Autodesk Fusion 360 part; units mm, degrees
sketch "Sketch1" plane through (0, 0, 0) normal (0, 0, 1) x (1, 0, 0)
  line L0 (-16.25, 11.25) -> (16.25, 11.25)
  line L1 (16.25, 11.25) -> (16.25, -11.25)
  line L2 (16.25, -11.25) -> (-16.25, -11.25)
  line L3 (-16.25, -11.25) -> (-16.25, 11.25)
  line L4 (-22.25, 13.25) -> (22.25, 13.25)
  line L5 (22.25, 13.25) -> (22.25, -13.25)
  line L6 (22.25, -13.25) -> (-22.25, -13.25)
  line L7 (-22.25, -13.25) -> (-22.25, 13.25)
  line L8 (-22.25, 13.25) -> (22.25, -13.25) construction
  line L9 (22.25, 13.25) -> (-22.25, -13.25) construction
  line L10 (-19.25, 7.5) -> (-19.25, -7.5) construction
  line L11 (-22.25, 0) -> (-16.25, 0) construction
  line L12 (16.25, 0) -> (22.25, 0) construction
  line L13 (19.25, 7.5) -> (19.25, -7.5) construction
  circle A0 centre (-19.25, 7.5) radius 1
  circle A1 centre (-19.25, -7.5) radius 1
  circle A2 centre (19.25, -7.5) radius 1
  circle A3 centre (19.25, 7.5) radius 1
  point P0 (-19.25, 0)
  point P1 (-19.25, 0)
  point P2 (19.25, 0)
  point P3 (19.25, 0)
  dimension "d1" = 32.5
  dimension "d2" = 22.5
  dimension "d3" = 2
  dimension "d4" = 6
  dimension "d21" = 6
  dimension "d22" = 2
  dimension "d23" = 15
  dimension "d24" = 2
extrude "Extrude1" add sketch "Sketch1" against normal blind 2 contours L0 L1 L2 L3 | L4 L5 L6 L7
extrude "Extrude2" add sketch "Sketch1" along normal blind 10
sketch "Sketch2" plane through (0, 0, 0) normal (0, 0, 1) x (-1, 0, 0)
  line L0 (-16.25, 11.25) -> (-16.25, -11.25)
  line L1 (-16.25, -11.25) -> (16.25, -11.25)
  line L2 (16.25, -11.25) -> (16.25, 11.25)
  line L3 (16.25, 11.25) -> (-16.25, 11.25)
  line L4 (12.5, 9) -> (12.5, -9) construction
  line L5 (12.5, -9) -> (-9.5, -9) construction
  line L6 (-9.5, 9) -> (12.5, 9) construction
  line L7 (-9.5, -9) -> (-9.5, 9) construction
  line L8 (12.5, -9) -> (-9.5, 9) construction
  line L9 (12.5, 9) -> (-9.5, -9) construction
  line L10 (14.375, -11.25) -> (10.625, -11.25)
  line L11 (10.625, -11.25) -> (10.625, -6.75)
  line L12 (10.625, -6.75) -> (14.375, -6.75)
  line L13 (14.375, -6.75) -> (14.375, -11.25)
  line L14 (14.375, -11.25) -> (10.625, -6.75) construction
  line L15 (10.625, -11.25) -> (14.375, -6.75) construction
  line L16 (-7.625, -11.25) -> (-11.375, -11.25)
  line L17 (-11.375, -11.25) -> (-11.375, -6.75)
  line L18 (-11.375, -6.75) -> (-7.625, -6.75)
  line L19 (-7.625, -6.75) -> (-7.625, -11.25)
  line L20 (-7.625, -11.25) -> (-11.375, -6.75) construction
  line L21 (-11.375, -11.25) -> (-7.625, -6.75) construction
  line L22 (14.375, 11.25) -> (10.625, 11.25)
  line L23 (10.625, 11.25) -> (10.625, 6.75)
  line L24 (10.625, 6.75) -> (14.375, 6.75)
  line L25 (14.375, 6.75) -> (14.375, 11.25)
  line L26 (14.375, 11.25) -> (10.625, 6.75) construction
  line L27 (10.625, 11.25) -> (14.375, 6.75) construction
  line L28 (-11.375, 11.25) -> (-7.625, 11.25)
  line L29 (-7.625, 11.25) -> (-7.625, 6.75)
  line L30 (-7.625, 6.75) -> (-11.375, 6.75)
  line L31 (-11.375, 6.75) -> (-11.375, 11.25)
  line L32 (-11.375, 11.25) -> (-7.625, 6.75) construction
  line L33 (-7.625, 11.25) -> (-11.375, 6.75) construction
  circle A0 centre (12.5, -9) radius 0.875
  circle A1 centre (-9.5, -9) radius 0.875
  circle A2 centre (-9.5, 9) radius 0.875
  circle A3 centre (12.5, 9) radius 0.875
  circle A4 centre (-9.5, 0) radius 4.5
  point P0 (1.5, 0)
  point P1 (12.5, -9)
  point P2 (-9.5, -9)
  point P3 (12.5, 9)
  point P4 (-9.5, 9)
  dimension "d9" = 18
  dimension "d10" = 22
  dimension "d11" = 1.5
  dimension "d12" = 3.75
  dimension "d13" = 1.75
  dimension "d16" = 9
extrude "Extrude3" add sketch "Sketch2" along normal blind 7 contours L3 L28 L29 L30 L31 | L1 L16 L17 L18 L19 | L3 L22 L23 L24 L25 | L1 L10 L11 L12 L13 | A0 | A1 | A2 | A3
extrude "Extrude4" cut sketch "Sketch2" against normal through all contours A4
sketch "Sketch3" plane through (0, 0, -2) normal (0, 0, -1) x (1, 0, 0)
  circle A0 centre (9.5, 0) radius 4.5
  circle A1 centre (19.25, -7.5) radius 1
  circle A2 centre (-19.25, 7.5) radius 1
  circle A3 centre (19.25, 7.5) radius 1
  circle A4 centre (-19.25, -7.5) radius 1
  line L0 (22.25, 13.25) -> (-22.25, 13.25)
  line L1 (-22.25, 13.25) -> (-22.25, -13.25)
  line L2 (-22.25, -13.25) -> (22.25, -13.25)
  line L3 (22.25, -13.25) -> (22.25, 13.25)
  circle A5 centre (-19.25, 7.5) radius 2
  circle A6 centre (-19.25, -7.5) radius 2
  circle A7 centre (19.25, -7.5) radius 2
  circle A8 centre (19.25, 7.5) radius 2
  dimension "d25" = 4
extrude "Extrude5" cut sketch "Sketch3" against normal blind 4 contours A5 | A6 | A7 | A8
fillet "Fillet1" radius 2 4 edges at (22.25, 13.25, 4) (-22.25, 13.25, 4) (-22.25, -13.25, 4) (22.25, -13.25, 4)
chamfer "Chamfer1" distance 1 angle 45 8 edges at (0, -13.25, -2) (-21.6642, -12.6642, -2) (-22.25, 0, -2) (-21.6642, 12.6642, -2) (0, 13.25, -2) (21.6642, 12.6642, -2) (22.25, 0, -2) (21.6642, -12.6642, -2)
equation "d21 = d4"
equation "d22 = d3"
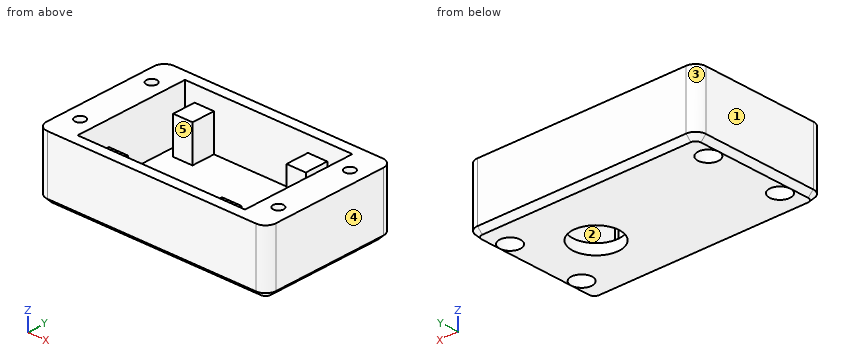
The listing builds one solid part. Answer for the finished solid, in the listing's coordinates (mm). Face numbers are marked on the shaded views. A direction names the side the tool comes from. Coordinates: 2 decimals unless noted, no trailing zeros. Loops run counter-clockwise (first coordinate to the right, second up) from the corner with the lowest first, then second, coordinate; pieces in that order, holes last. Notation, with made-up numbers: (15.5, 35.25) - (40.5, 35.25) arc R33 cw to (40.5, 66.25) - close; hole circle Ø2 at (-26.75, 75.5). An arc over 180 degrees is marked (long way). Use a Markdown table: item, result. Add a question column.
1) For the marked faces 4 and 5, determine the directions among +Z, -Z, +X, -X, +Y, -Y from which every point of the face is accessible in a straight line to the end or side of a thin tool.
2) Find the intervals of material crossed by line 1 (X direction, y = -10, z = 4.75) (3 decimals); line 2 (X direction, y = -7.5, z = 0.25) (3 decimals); line 3 (Y direction, x = 19.25, z = 7.75), in increasing order.
3) Given pin 1 (10 mm diameter, centred on x = 2.5, y = 4.5, fed in from +Z); pin 2 (2.5 mm diameter, centred on x = -19.25, y = 7.5, fed in from -Z); pin 3 (3 mm diameter, centred on x = 19.25, y = -7.5, fed in from +Z), each flat-ended and moving along its own axis, determine where each tip first touches the part or whether it passes through.
4) The part is cut by section B-B, the plane y = 7.5. State how many separate pieces and enclosed holes the cut face has, and give its area (4 significant figures).
5) The part is cut by section D-D, the plane x = 9.5. Give the vertices of the cut face in (y, z), and give its area (3 significant figures).
6) The mould has two halves that part along Y. Classify the marked faces 1, 2 and 3: released by +Y, released by -Y, zero draft, split by the parting line, or undercut.
7) The part is cut by section A-A, the plane x = -19.25. Give the vertices of the cut face in (y, z), and give its area (3 significant figures).
Here are the results:
| question | item | result |
|---|---|---|
| 1 | face 4 | +Z, -Z, +X, +Y, -Y |
| 1 | face 5 | +Z |
| 2 | line 1 | x = -22.25 to -16.25, -14.375 to -10.625, 7.625 to 11.375, 16.25 to 22.25 |
| 2 | line 2 | x = -22.25 to -21.25, -17.25 to -16.25, -14.375 to -10.625, 7.625 to 11.375, 16.25 to 17.25, 21.25 to 22.25 |
| 2 | line 3 | y = -13.25 to -8.5, -6.5 to 6.5, 8.5 to 13.25 |
| 3 | pin 1 | stops at z = 0 |
| 3 | pin 2 | stops at z = 2 |
| 3 | pin 3 | stops at z = 10 |
| 4 | separate pieces | 3 |
| 4 | enclosed holes | 0 |
| 4 | area | 196.5 mm^2 |
| 5 | outline | (-13.25, -1) - (-12.25, -2) - (-4.5, -2) - (-4.5, 0) - (-6.75, 0) - (-6.75, 7) - (-11.25, 7) - (-11.25, 10) - (-13.25, 10) - close; (4.5, -2) - (12.25, -2) - (13.25, -1) - (13.25, 10) - (11.25, 10) - (11.25, 7) - (6.75, 7) - (6.75, 0) - (4.5, 0) - close |
| 5 | area | 137 mm^2 |
| 6 | face 1 | zero draft |
| 6 | face 2 | undercut |
| 6 | face 3 | released by +Y |
| 7 | outline | (-13.25, -1) - (-12.25, -2) - (-9.5, -2) - (-9.5, 2) - (-8.5, 2) - (-8.5, 10) - (-13.25, 10) - close; (-6.5, 2) - (-5.5, 2) - (-5.5, -2) - (5.5, -2) - (5.5, 2) - (6.5, 2) - (6.5, 10) - (-6.5, 10) - close; (8.5, 2) - (9.5, 2) - (9.5, -2) - (12.25, -2) - (13.25, -1) - (13.25, 10) - (8.5, 10) - close |
| 7 | area | 253 mm^2 |
